The listing builds one solid part. Answer for the finished solid, in the listing's coordinates (mm). Face numbers are marked on the shaded views. A direction names the side the tool comes from. Give positions to 0.01 mm unless a question says otherwise; leave off trailing zeros. Loops run counter-clockwise (first coordinate to the right, second up) from the corner with the lowest first, then second, coordinate; pieces in that order, holes last. Notation, with made-up numbers: M -39,72 L -13,72 A24 cw -13,111 Z; hole C -39,23.5 d4. An arc over 180 degrees is marked long. One line per item, written item: value. Start each with the question number.
Q1. A cutting plane is placed at B-B, the plane y = 7. Determine the outline of the cut face in (x, z), and give its area (3 significant figures).
Q2. Flat-ended cylindrical pins translate along their axes: pin 1 (2.5 mm diameter, centred on x = 5, y = 12, fed in from +Z); pin 2 (4 mm diameter, centred on x = 3.5, z = -9, fed in from +Y); pin 3 (3 mm diameter, centred on x = 4, z = -18, fed in from +Y); pin 4 (2 mm diameter, centred on y = 12, z = -18.5, fed in from +X). Find the tip coordinate at first contact, or state that the pin passes through.
Q3. A cutting plane is placed at C-C, the plane z = -12. Determine the outline of the cut face in (x, y), and give its area (3 significant figures).
Q4. A cutting plane is placed at D-D, the plane x = 1. Determine the outline of the cut face in (y, z), and give its area (3 significant figures).
Q5. A cutting plane is placed at A-A, the plane x = 4. Determine the outline of the cut face in (y, z).
Q6. For the marked faces 4 and 5, determine the directions among +Z, -Z, +X, -X, +Y, -Y from which every point of the face is accessible in a straight line to the end or side of a thin tool.
Q7. Consider L1, parallel to Z at x = 4, y = 2.2; L2, parallel to X at y = 2.25, z = -18; L3, parallel to Z at x = 3, y = 27. Determine where each line is inside the solid, lowest interval first.
Q8. The mould has two halves that part along Z. Classify the marked faces 1, 2 and 3: +Z half, -Z half, draft (parallel to the pull), parting line (faces both ways), or undercut.
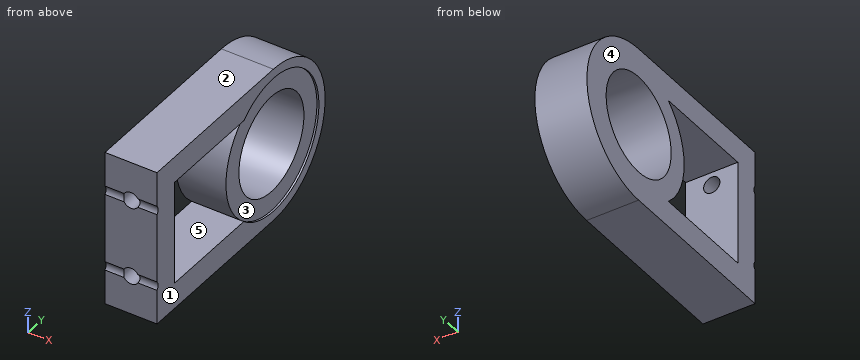
Autodesk Inventor part; units mm, degrees
ref_plane "YZ Plane" through (0, 0, 0) normal (1, 0, 0) x (0, 1, 0)
ref_plane "XZ Plane" through (0, 0, 0) normal (0, 1, 0) x (-1, 0, 0)
ref_plane "XY Plane" through (0, 0, 0) normal (0, 0, 1) x (1, 0, 0)
sketch "스케치1" plane through (0, 0, 0) normal (1, 0, 0) x (0, 1, 0)
  line L0 (0, 0) -> (27, 0)
  line L1 (27, -24) -> (0, -24)
  line L2 (0, -24) -> (0, 0)
  circle A0 centre (27, -12) radius 7.55
  arc A1 (27, -24) -> (27, 0) centre (27, -12) ccw
  dimension "d2" = 15.1
  dimension "d3" = 12
  dimension "d4" = 27
  dimension "d8" = 24
extrude "돌출2" add sketch "스케치1" along normal blind 8
sketch "스케치2" plane through (8, 0, 0) normal (1, 0, 0) x (0, 0, -1)
  circle A0 centre (12, 27) radius 7.55
  line L0 (0, 27) -> (0, 0)
  line L1 (0, 0) -> (24, 0)
  line L2 (24, 0) -> (24, 27)
  arc A1 (24, 27) -> (0, 27) centre (12, 27) ccw
  arc A2 (4, 20.1223) -> (20, 20.1223) centre (12, 27) ccw
  line L3 (4, 4) -> (4, 20.1223)
  line L4 (20, 20.1223) -> (20, 4)
  line L5 (20, 4) -> (4, 4)
  dimension "d12" = 3
  dimension "d13" = 4
extrude "돌출3" cut sketch "스케치2" against normal blind 8 contours A2 L4 L5 L3
sketch "스케치3" plane through (0, 0, -24) normal (0, -1, 0) x (1, 0, 0)
  circle A0 centre (4, 18) radius 1.25
  circle A1 centre (4, 6) radius 1.25
  line L0 (8, 24) -> (8, 0)
  line L1 (0, 24) -> (8, 24)
  line L2 (0, 0) -> (8, 0)
  dimension "d16" = 2.5
  dimension "d17" = 2.5
  dimension "d18" = 4
  dimension "d19" = 4
  dimension "d20" = 6
  dimension "d21" = 6
extrude "돌출4" cut sketch "스케치3" against normal blind 8
sketch "스케치4" plane through (8, 0, 0) normal (1, 0, 0) x (0, 0, -1)
  line L0 (4.75, 4) -> (7.25, 4)
  line L1 (7.25, 0) -> (4.75, 0)
  line L2 (16.75, 4) -> (19.25, 4)
  line L3 (19.25, 0) -> (16.75, 0)
  arc A0 (6.6614, 0) -> (5.3386, 0) centre (6, -0.75) ccw
  arc A1 (18.6614, 0) -> (17.3386, 0) centre (18, -0.75) ccw
  line L4 (0, 0) -> (24, 0)
  dimension "d24" = 2
  dimension "d25" = 2
extrude "돌출5" cut sketch "스케치4" against normal blind 8
sketch "스케치5" plane through (8, 0, 0) normal (1, 0, 0) x (0, 0, -1)
  arc A0 (6.6614, 0) -> (5.3386, 0) centre (6, -0.75) ccw
  line L0 (6.6614, 0) -> (17.3386, 0)
  arc A1 (18.6614, 0) -> (17.3386, 0) centre (18, -0.75) ccw
  line L1 (18.6614, 0) -> (24, 0)
  line L2 (24, 0) -> (24, 27)
  arc A2 (24, 27) -> (0, 27) centre (12, 27) ccw
  line L3 (0, 27) -> (0, 0)
  line L4 (0, 0) -> (5.3386, 0)
  circle A3 centre (12, 27) radius 7.55
  line L5 (20, 4) -> (4, 4)
  line L6 (4, 4) -> (4, 20.1223)
  arc A4 (4, 20.1223) -> (20, 20.1223) centre (12, 27) ccw
  line L7 (20, 20.1223) -> (20, 4)
  circle A5 centre (12, 27) radius 10.55
extrude "돌출6" cut sketch "스케치5" against normal blind 0.3 contours A4 A5
properties part number "베어링받침대" material "알루미늄 6061"
Answer block:
1. outline: M 0,-24 L 8,-24 L 8,-20 L 0,-20 Z; M 0,-4 L 8,-4 L 8,0 L 0,0 Z
1. area: 64.0 mm^2
2. pin 1: z = 0
2. pin 2: y = 38.96
2. pin 3: y = 38.12
2. pin 4: through
3. outline: M 0,0 L 8,0 L 8,4 L 0,4 Z; M 0,16.45 L 7.7,16.45 L 7.7,19.45 L 0,19.45 Z; M 0,34.55 L 7.7,34.55 L 7.7,37.55 L 8,37.55 L 8,39 L 0,39 Z
3. area: 89.8 mm^2
4. outline: M 0,-24 L 27,-24 A12 ccw 27,0 L 0,0 L 0,-5.34 A1 cw 0,-6.66 L 0,-17.34 A1 cw 0,-18.66 Z; hole M 4,-20 L 20.12,-20 A10.55 cw 20.12,-4 L 4,-4 Z; hole C 27,-12 d15.1
4. area: 477 mm^2
5. outline: M 0,-24 L 27,-24 A12 ccw 27,0 L 0,0 L 0,-4.75 L 4,-4.75 L 4,-4 L 20.12,-4 A10.55 ccw 20.12,-20 L 4,-20 L 4,-19.25 L 0,-19.25 Z; M 0,-16.75 L 4,-16.75 L 4,-7.25 L 0,-7.25 Z; hole C 27,-12 d15.1
6. face 4: +Z, -Z, -X, +Y, -Y
6. face 5: +X, -X
7. L1: -24 to -19.25, -16.75 to -7.25, -4.75 to 0
7. L2: 0 to 2.75, 5.25 to 8
7. L3: -24 to -19.55, -4.45 to 0
8. face 1: draft
8. face 2: +Z half
8. face 3: undercut
